from build123d import *

# Parameters (mm, degrees)
F2_R     = 2.5
F3_DEPTH = 25
F4_R     = 2
F5_R     = 9
F6_R     = 10
F7_R     = 7


with BuildPart() as f1:
    # F0 (on Front) → F1 (revolve)
    with BuildSketch(Plane.XZ):
        Polygon((0, 24), (0, 0), (8.1, 0), (8.1, 12), (11.974087, 19.68414), (14.15, 19.68414), (14.15, 24), align=None)
    revolve(axis=Axis((0, 0, 12), (0, 0, 1)))

    # F2 (on face) → F3 (cut)
    with BuildSketch(Plane(origin=(0, 0, 0), x_dir=(1, 0, 0), z_dir=(0, 0, -1))):
        Circle(F2_R)
    extrude(amount=-F3_DEPTH, mode=Mode.SUBTRACT)

    # F4
    f4_edges = [f1.edges().sort_by_distance(p)[0] for p in [
        (-14.15, 0, 24),
        (-14.15, 0, 19.68414),
    ]]
    fillet(f4_edges, radius=F4_R)

    # F5
    f5_edges = [f1.edges().sort_by_distance(p)[0] for p in [
        (-11.974087, 0, 19.68414),
    ]]
    fillet(f5_edges, radius=F5_R)

    # F6
    f6_edges = [f1.edges().sort_by_distance(p)[0] for p in [
        (-8.1, 0, 12),
    ]]
    fillet(f6_edges, radius=F6_R)

    # F7
    f7_edges = [f1.edges().sort_by_distance(p)[0] for p in [
        (-2.5, 0, 24),
    ]]
    fillet(f7_edges, radius=F7_R)


solid = f1.part
CAD build for the part. Positions are in the model's coordinates, mm. Give positions to 0.01 mm unless a question says otherwise; leave off trailing zeros. Order: outer loops, then holes, each group sorted by start corner. A loop starts at its lowest first (then second) coordinate and runs counter-clockwise, first axis right, second up. Notation, with made-up numbers: (53.25, -17.5) - (83.25, -17.5) arc R24 cw to (83.25, 14.5) - close; hole circle Ø8 at (41.5, 15). An arc over 180 degrees is marked (long way). Answer in a Markdown table with one row per item.
1. Flat gauge pins, fed straight in: pin 1 (4 mm diameter, centred on y = -9.5, z = 2.5, fed in from -X); pin 2 (3 mm diameter, centred on y = -2, z = 4, fed in from -X); pin 3 (10 mm diameter, centred on x = 7, z = 2.5, fed in from +Y). Where does each tip first touch, or does it go through?
Data:
| item | result |
|---|---|
| pin 1 | stops at x = -3.06 |
| pin 2 | stops at x = -8.08 |
| pin 3 | stops at y = 7.85 |
2. Probe probe 1 along X at (y, z) = (0, 8.75); probe 2 along Y at (x, z) = (-1, 15.5). List the from-to ranges inside material, lowest first. Write a range as [from, to].
Data:
| item | result |
|---|---|
| probe 1 | x = [-8.1, -2.5], [2.5, 8.1] |
| probe 2 | y = [-9.81, -2.29], [2.29, 9.81] |
3. Pull direction X, two halves, no side cores. Call faces 1 (the cylindrical face through (7.726, 2.433, 4.878)), 2 (the cylindrical face through (-0.54, 2.44, 8.38)), 3 (the flat face through (2, -2, 0)): pulls with the +X half, pulls with the -X half, needs draft (parallel to the pull), parting line crosses it, or undercut.
Data:
| item | result |
|---|---|
| face 1 | parting line crosses it |
| face 2 | undercut |
| face 3 | needs draft |
4. Saw through at A-A, the plane z = 4. Give the cut face in (x, y), plus the area to 3 significant figures.
Data:
| item | result |
|---|---|
| outline | circle Ø16.2 at (0, 0); hole circle Ø5 at (0, 0) |
| area | 186 mm² |
